from build123d import *

# Parameters (mm, degrees)
SKETCH1_R           = 3
SKETCH1_R_2         = 16
BOSS_EXTRUDE1_DEPTH = 3
SKETCH3_R           = 30
SKETCH3_R_2         = 21
BOSS_EXTRUDE3_DEPTH = 3.5
SKETCH4_R           = 3
BOSS_EXTRUDE4_DEPTH = 3.5
SKETCH5_R           = 3
SKETCH5_R_2         = 21
CUT_EXTRUDE1_DEPTH  = 0.5


with BuildPart() as part:
    # Sketch1 → Boss-Extrude1 (new body)
    with BuildSketch(Plane.XY):
        with BuildLine():
            Line((-65, 20), (-65, -20))
            Line((-65, -20), (-4.730882844, -29.624630757))
            ThreePointArc((-4.730882844, -29.624630757), (0, -30), (4.730882844, -29.624630757))
            Line((4.730882844, -29.624630757), (65, -20))
            Line((65, -20), (65, 20))
            Line((65, 20), (4.730882844, 29.624630757))
            ThreePointArc((4.730882844, 29.624630757), (0, 30), (-4.730882844, 29.624630757))
            Line((-4.730882844, 29.624630757), (-65, 20))
        make_face()
        with Locations((56, 0)):
            Circle(SKETCH1_R, mode=Mode.SUBTRACT)
        with Locations((42, 0)):
            Circle(SKETCH1_R, mode=Mode.SUBTRACT)
        with Locations((-56, 0)):
            Circle(SKETCH1_R, mode=Mode.SUBTRACT)
        with Locations((-42, 0)):
            Circle(SKETCH1_R, mode=Mode.SUBTRACT)
        Circle(SKETCH1_R_2, mode=Mode.SUBTRACT)
    extrude(amount=BOSS_EXTRUDE1_DEPTH)

    # Sketch3 → Boss-Extrude3 (add)
    with BuildSketch(Plane(origin=(0, 0, 0), x_dir=(-1, 0, 0), z_dir=(0, 0, -1))):
        Circle(SKETCH3_R)
        Circle(SKETCH3_R_2, mode=Mode.SUBTRACT)
    extrude(amount=BOSS_EXTRUDE3_DEPTH)

    # Sketch4 → Boss-Extrude4 (add)
    with BuildSketch(Plane(origin=(0, 0, 0), x_dir=(-1, 0, 0), z_dir=(0, 0, -1))):
        with BuildLine():
            Line((4.730882844, -29.624630757), (65, -20))
            Line((65, -20), (65, 20))
            Line((65, 20), (4.730882844, 29.624630757))
            ThreePointArc((4.730882844, 29.624630757), (30, 0), (4.730882844, -29.624630757))
        make_face()
        with Locations((56, 0)):
            Circle(SKETCH4_R, mode=Mode.SUBTRACT)
        with Locations((42, 0)):
            Circle(SKETCH4_R, mode=Mode.SUBTRACT)
        with BuildLine():
            Line((-4.730882844, 29.624630757), (-65, 20))
            Line((-65, 20), (-65, -20))
            Line((-65, -20), (-4.730882844, -29.624630757))
            ThreePointArc((-4.730882844, -29.624630757), (-30, 0), (-4.730882844, 29.624630757))
        make_face()
        with Locations((-42, 0)):
            Circle(SKETCH4_R, mode=Mode.SUBTRACT)
        with Locations((-56, 0)):
            Circle(SKETCH4_R, mode=Mode.SUBTRACT)
    extrude(amount=BOSS_EXTRUDE4_DEPTH)

    # Sketch5 → Cut-Extrude1 (cut)
    with BuildSketch(Plane(origin=(0, 0, -3.5), x_dir=(-1, 0, 0), z_dir=(0, 0, -1))):
        with BuildLine():
            Line((-4.730882844, 29.624630757), (-65, 20))
            Line((-65, 20), (-65, -20))
            Line((-65, -20), (-4.730882844, -29.624630757))
            ThreePointArc((-4.730882844, -29.624630757), (0, -30), (4.730882844, -29.624630757))
            Line((4.730882844, -29.624630757), (65, -20))
            Line((65, -20), (65, 20))
            Line((65, 20), (4.730882844, 29.624630757))
            ThreePointArc((4.730882844, 29.624630757), (0, 30), (-4.730882844, 29.624630757))
        make_face()
        with Locations((56, 0)):
            Circle(SKETCH5_R, mode=Mode.SUBTRACT)
        with Locations((42, 0)):
            Circle(SKETCH5_R, mode=Mode.SUBTRACT)
        Circle(SKETCH5_R_2, mode=Mode.SUBTRACT)
        with Locations((-42, 0)):
            Circle(SKETCH5_R, mode=Mode.SUBTRACT)
        with Locations((-56, 0)):
            Circle(SKETCH5_R, mode=Mode.SUBTRACT)
    extrude(amount=-CUT_EXTRUDE1_DEPTH, mode=Mode.SUBTRACT)


solid = part.part
Build history of the part. All positions in model axes, mm. A direction names the side the tool comes from. Coordinates: 2 decimals unless noted, no trailing zeros. Write each loop counter-clockwise with the first axis right and the second up, starting at its lowest first coordinate (ties: lowest second). Pieces come first, ordered by that corner, then holes.
(1) Cut at A-A on z = -1.15. List the corners of the cut face in (x, y), and give its area (3 significant figures).
(2) Cut at C-C on y = 7. List the corners of the cut face in (x, z).
(3) Cut at D-D on x = -42. List the corners of the cut face in (y, z).
(4) Cut at B-B on x = -55. List the corners of the cut face in (y, z).
(5) Pin check, flat tips, straight feed: pin 1 Ø3.5 at (x, y) = (56, 0) entering from +Z; pin 2 Ø12.5 at (x, y) = (-10.5, 3.5) entering from -Z; pin 3 Ø3 at (x, z) = (27, 0) entering from +Y; pin 4 Ø3 at (x, z) = (19, 2) entering from +Y. Stop position of each tip, or through.
(6) 3-axis set-ups, long thin cutter, end or side, ignore diameter. For faces 4 (the flat face through (-4.8, -15.5, 0)), 5 (the flat face through (35.287, 24.745, -0.042)): which of +Z, -Z, +X, -X, +Y, -Y reach the whole face in a straight line?
(7) Drill centre lines: line 1 (Y direction, x = 0, z = 1.5); line 2 (X direction, y = -2.5, z = 2.1); line 3 (Y direction, x = -16.5, z = -0.7). Where is each one in solid material? Low to high.
(8) Mould opens along X. For faces 1 (the flat face through (15, -20, -3)), 2 (the flat face through (-35.287, 24.745, 0.042)), 3 (the cylindrical face through (-20.03, 6.31, -1.48)) say: pulls with the +X half, pulls with the -X half, needs draft (parallel to the pull), parting line crosses it, or undercut.
Working result:
1. outline: (-65, -20) - (-4.73, -29.62) arc R30 ccw to (4.73, -29.62) - (65, -20) - (65, 20) - (4.73, 29.62) arc R30 ccw to (-4.73, 29.62) - (-65, 20) - close; hole circle Ø6 at (-56, 0); hole circle Ø6 at (-42, 0); hole circle Ø42 at (0, 0); hole circle Ø6 at (42, 0); hole circle Ø6 at (56, 0)
1. area: 5,050 mm2
2. outline: (-65, -3) - (-19.8, -3) - (-19.8, 0) - (-14.39, 0) - (-14.39, 3) - (-65, 3) - close; (14.39, 0) - (19.8, 0) - (19.8, -3) - (65, -3) - (65, 3) - (14.39, 3) - close
3. outline: (-23.67, -3) - (-3, -3) - (-3, 3) - (-23.67, 3) - close; (3, -3) - (23.67, -3) - (23.67, 3) - (3, 3) - close
4. outline: (-21.6, -3) - (-2.83, -3) - (-2.83, 3) - (-21.6, 3) - close; (2.83, -3) - (21.6, -3) - (21.6, 3) - (2.83, 3) - close
5. pin 1: passes through
5. pin 2: stops at z = 0
5. pin 3: stops at y = 26.31
5. pin 4: stops at y = 27.59
6. face 4: -Z
6. face 5: +Z, -Z, +X, +Y
7. line 1: y = -30 to -16, 16 to 30
7. line 2: x = -65 to -57.66, -54.34 to -43.66, -40.34 to -15.8, 15.8 to 40.34, 43.66 to 54.34, 57.66 to 65
7. line 3: y = -27.75 to -12.99, 12.99 to 27.75
8. face 1: needs draft
8. face 2: pulls with the -X half
8. face 3: undercut
